Autodesk Inventor part; units mm, degrees
ref_plane "YZ Plane" through (0, 0, 0) normal (1, 0, 0) x (0, 1, 0)
ref_plane "XZ Plane" through (0, 0, 0) normal (0, 1, 0) x (-1, 0, 0)
ref_plane "XY Plane" through (0, 0, 0) normal (0, 0, 1) x (1, 0, 0)
sketch "スケッチ1" plane through (0, 0, 0) normal (0, 0, 1) x (1, 0, 0)
  line L0 (-9.05, -7) -> (9.05, -7)
  line L1 (9.05, -7) -> (9.05, 7)
  line L2 (9.05, 7) -> (-9.05, 7)
  line L3 (-9.05, 7) -> (-9.05, -7)
  line L4 (-9.05, -7) -> (9.05, 7) construction
  line L5 (9.05, -7) -> (-9.05, 7) construction
  point P0 (0, 0)
  dimension "d1" = 14
  dimension "d2" = 18.1
extrude "押し出し1" add sketch "スケッチ1" along normal blind 42.8
sketch "スケッチ2" plane through (0, 0, 42.8) normal (0, 0, 1) x (1, 0, 0)
  line L0 (-9.05, 7) -> (-9.05, -7)
  line L1 (-9.05, 7) -> (-7, 7)
  line L2 (-7, 7) -> (-9.05, -2)
  line L3 (9.05, 7) -> (-9.05, 7)
  line L4 (-9.05, 7) -> (-9.05, -2)
  line L5 (9.05, -7) -> (9.05, 7)
  line L6 (9.05, 7) -> (9.05, -2)
  line L7 (9.05, -2) -> (7, 7)
  line L8 (7, 7) -> (9.05, 7)
  line L9 (-9.05, -7) -> (9.05, -7)
  point P0 (0, 0)
  dimension "d5" = 14
  dimension "d6" = 5
extrude "押し出し2" cut sketch "スケッチ2" against normal through all contours L1 L2 L0 | L3 L5 L7
sketch "スケッチ3" plane through (-7, 7, 0) normal (0, 1, 0) x (1, 0, 0)
  line L0 (-2.05, 0) -> (-2.05, -42.8)
  line L1 (16.05, 0) -> (16.05, -42.8)
  line L2 (-2.05, -38.8) -> (16.05, -38.8)
  line L3 (16.05, -38.8) -> (16.05, -4)
  line L4 (16.05, -4) -> (-2.05, -4)
  line L5 (-2.05, -4) -> (-2.05, -38.8)
  line L6 (14, 0) -> (0, 0)
  line L7 (14, -42.8) -> (0, -42.8)
  point P0 (7, 0)
  dimension "d9" = 4
  dimension "d10" = 4
extrude "押し出し3" cut sketch "スケッチ3" against normal blind 8
sketch "スケッチ4" plane through (-7, 7, 4) normal (0, 0, 1) x (1, 0, 0)
  circle A0 centre (7, -4.45) radius 8.25
  line L0 (-2.05, -14) -> (16.05, -14)
  point P0 (7, -7)
  dimension "d13" = 16.5
  dimension "d14" = 17.8
extrude "押し出し4" cut sketch "スケッチ4" along normal up to surface (34.8 mm away)
sketch "スケッチ5" plane through (-7, 7, 0) normal (0, 1, 0) x (1, 0, 0)
  line L0 (2.1, -3) -> (11.9, -3)
  line L1 (11.9, -3) -> (11.9, -1)
  line L2 (11.9, -1) -> (2.1, -1)
  line L3 (2.1, -1) -> (2.1, -3)
  line L4 (2.1, -3) -> (11.9, -1) construction
  line L5 (11.9, -3) -> (2.1, -1) construction
  line L6 (14, -4) -> (14, 0)
  line L7 (14, 0) -> (0, 0)
  point P0 (7, 0)
  point P1 (7, -2)
  point P2 (7, -2)
  point P3 (14, -2)
  point P4 (7, -2)
  point P5 (7, 0)
  dimension "d17" = 2
  dimension "d18" = 9.8
extrude "押し出し5" cut sketch "スケッチ5" against normal blind 13
Input: part model. Units: mm. Frame: model coordinates. A direction names the side the tool comes from. Give positions to 0.01 mm unless a question says otherwise; leave off trailing zeros. Loops run counter-clockwise (first coordinate to the right, second up) from the corner with the lowest first, then second, coordinate; pieces in that order, holes last. Notation, with made-up numbers: (37, -31.75) -> (51, -31.75) arc R31 ccw to (51, 4.25) -> close; hole circle Ø6 at (66.25, -7.75). An arc over 180 degrees is marked (long way). Use a Markdown table: item, result.
Q1. Section query C-C, the plane z = 17.5. Return the cut outline in (x, y), plus the area to 3 significant figures.
Entries:
| item | result |
|---|---|
| outline | (-9.05, -7) -> (9.05, -7) -> (9.05, -2) -> (8.82, -1) -> (7.45, -1) arc R8.25 cw to (-7.45, -1) -> (-8.82, -1) -> (-9.05, -2) -> close |
| area | 58.2 mm² |
Q2. Pull-direction query (Z, two-part tool) for faces 1 (the flat face through (9.05, -5, 21)), 2 (the flat face through (-8, -1, 21)), 3 (the flat face through (0, 0, 42.8)); classes: pulls with the +Z half, pulls with the -Z half, needs draft (parallel to the pull), parting line crosses it, or undercut.
Entries:
| item | result |
|---|---|
| face 1 | needs draft |
| face 2 | undercut |
| face 3 | pulls with the +Z half |
Q3. Ray query, probe 1 along Z at (x, y) = (-3.75, 5.75); probe 2 along Z at (x, y) = (-6.25, 4.75); probe 3 along X at (y, z) = (-3.5, 22.5). Return the intervals inside material, ascending. Write a range as from..to.
Entries:
| item | result |
|---|---|
| probe 1 | z = 0..1, 3..4, 38.8..42.8 |
| probe 2 | z = 0..4, 38.8..42.8 |
| probe 3 | x = -9.05..-5.61, 5.61..9.05 |
Q4. Section query A-A, the plane y = 2.5. Return the cut outline in (x, z) (3 decimals).
Entries:
| item | result |
|---|---|
| outline | (-8.025, 0) -> (8.025, 0) -> (8.025, 4) -> (-8.025, 4) -> close; (-8.025, 38.8) -> (8.025, 38.8) -> (8.025, 42.8) -> (-8.025, 42.8) -> close; hole (-4.9, 1) -> (4.9, 1) -> (4.9, 3) -> (-4.9, 3) -> close |
Q5. Access query for faces 4 (the flat face through (0, 0, 0)), 5 (the flat face through (-4.9, 1, 2)), 6 (the flat face through (8, -1, 21)). Directions: +Z, -Z, +X, -X, +Y, -Y. A direction counts if a zero-diameter tool reaches every point of the face in a straight line with its end or side. Return the directions, or none.
Entries:
| item | result |
|---|---|
| face 4 | -Z, +X, -X, +Y, -Y |
| face 5 | +Y |
| face 6 | +X, -X, +Y |
Q6. Section query B-B, the plane x = 0. Return the cut outline in (y, z), plus the area to 3 significant figures.
Entries:
| item | result |
|---|---|
| outline | (-7, 0) -> (7, 0) -> (7, 1) -> (-6, 1) -> (-6, 3) -> (7, 3) -> (7, 4) -> (-5.7, 4) -> (-5.7, 38.8) -> (7, 38.8) -> (7, 42.8) -> (-7, 42.8) -> close |
| area | 131 mm² |
Q7. Section query D-D, the plane y = 0.25. Return the cut outline in (x, z).
Entries:
| item | result |
|---|---|
| outline | (-8.54, 0) -> (8.54, 0) -> (8.54, 4) -> (-8.54, 4) -> close; (-8.54, 38.8) -> (8.54, 38.8) -> (8.54, 42.8) -> (-8.54, 42.8) -> close; hole (-4.9, 1) -> (4.9, 1) -> (4.9, 3) -> (-4.9, 3) -> close |
Q8. First-contact query: P1, Ø6, axis at y = 3.5, z = 35, coming from the +X side; P2, Ø1.6, axis at y = 3, z = 2, coming from the -X side; P3, Ø1.5, axis at x = -8, z = 24.5, coming from the +Y side; P4, Ø2, axis at x = -4, y = -0.5, coming from the -Z side. Flat tips, straight axial feed; report the tip coordinate or a pass-through.
Entries:
| item | result |
|---|---|
| P1 | passes through |
| P2 | stops at x = -8.09 |
| P3 | stops at y = -1 |
| P4 | stops at z = 0 |
